Work out the finished part from the listing and answer in its coordinate system (mm). Coordinates: 2 decimals unless noted, no trailing zeros. Write each loop counter-clockwise with the first axis right and the second up, starting at its lowest first coordinate (ties: lowest second). Pieces come first, ordered by that corner, then holes. Notation, with made-up numbers: (-21.5, 47) -> (-12.5, 47) arc R28 cw to (-12.5, 66) -> close; hole circle Ø4 at (-7.5, 55.5). An arc over 180 degrees is marked (long way). Write each question's results on one line, items separated by ' | '. Start each with the question number.
from build123d import *

# Parameters (mm, degrees)
F1_W     = 1447.8
F1_H     = 431.8
F1_W_2   = 25.4
F1_H_2   = 381
F2_DEPTH = 19.05


# Not quite as in the source:
# - a variable given as a bare number and used for a length is read in inches; the dataset says mm whatever the document's units were


with BuildPart() as f2:
    # F1 (on Front) → F2 (new body)
    with BuildSketch(Plane.XZ):
        Rectangle(F1_W, F1_H)
        Polygon((-698.5, -190.5), (-698.5, 190.5), (-254, 190.5), (-228.6, 190.5), (228.6, 190.5), (254, 190.5), (698.5, 190.5), (698.5, -190.5), (254, -190.5), (228.6, -190.5), (-228.6, -190.5), (-254, -190.5), align=None, mode=Mode.SUBTRACT)
        with Locations((-241.3, 0)):
            Rectangle(F1_W_2, F1_H_2)
        with Locations((241.3, 0)):
            Rectangle(F1_W_2, F1_H_2)
    extrude(amount=F2_DEPTH)


solid = f2.part
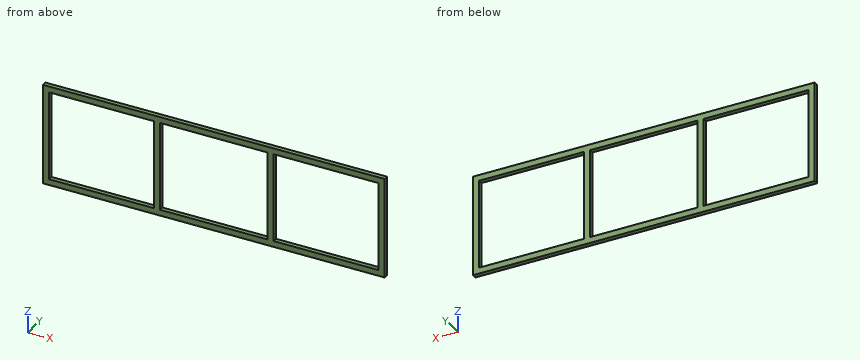
1. Find section C-C on y = -14.25. Give the vertices of the cut face in (x, z).
2. Find section A-A on x = 346. Give the vertices of the cut face in (y, z), and give its area (3 significant figures).
3. Find section B-B on z = 8. Give the vertices of the cut face in (x, y), and give its area (3 significant figures).
4. Find the intervals of material crossed by L1, parallel to X at y = -3, z = -51; L2, parallel to Z at x = -432, y = -7.75, in increasing order.
Ans:
1) outline: (-723.9, -215.9) -> (723.9, -215.9) -> (723.9, 215.9) -> (-723.9, 215.9) -> close; hole (-698.5, -190.5) -> (-254, -190.5) -> (-254, 190.5) -> (-698.5, 190.5) -> close; hole (-228.6, -190.5) -> (228.6, -190.5) -> (228.6, 190.5) -> (-228.6, 190.5) -> close; hole (254, -190.5) -> (698.5, -190.5) -> (698.5, 190.5) -> (254, 190.5) -> close
2) outline: (-19.05, -215.9) -> (0, -215.9) -> (0, -190.5) -> (-19.05, -190.5) -> close; (-19.05, 190.5) -> (0, 190.5) -> (0, 215.9) -> (-19.05, 215.9) -> close | area: 968 mm²
3) outline: (-723.9, -19.05) -> (-698.5, -19.05) -> (-698.5, 0) -> (-723.9, 0) -> close; (-254, -19.05) -> (-228.6, -19.05) -> (-228.6, 0) -> (-254, 0) -> close; (228.6, -19.05) -> (254, -19.05) -> (254, 0) -> (228.6, 0) -> close; (698.5, -19.05) -> (723.9, -19.05) -> (723.9, 0) -> (698.5, 0) -> close | area: 1,940 mm²
4) L1: x = -723.9 to -698.5, -254 to -228.6, 228.6 to 254, 698.5 to 723.9 | L2: z = -215.9 to -190.5, 190.5 to 215.9
